Model file for the job. Use its own axes, mm. A direction names the side the tool comes from. Coordinates: 2 decimals unless noted, no trailing zeros. Order: outer loops, then holes, each group sorted by start corner. A loop starts at its lowest first (then second) coordinate and runs counter-clockwise, first axis right, second up. Notation, with made-up numbers: (37.5, -11.75) -> (88.5, -11.75) arc R4 ccw to (88.5, -7.75) -> close; hole circle Ø9 at (13, -39). An arc over 180 degrees is marked (long way). Write item = value, one per line. Start each with the question number.
Q1. Flat gauge pins, fed straight in: pin 1 (10 mm diameter, centred on y = -6.5, z = -9, fed in from -X); pin 2 (7.5 mm diameter, centred on x = -20, y = -11, fed in from -Z); pin 3 (9 mm diameter, centred on x = 3.5, y = -40, fed in from +Z). Where does each tip first touch, or does it go through?
Q2. Cut at B-B, the plane y = -33.5. List the corners of the cut face in (x, z) (1 decimal), plus the area to 3 significant figures.
Q3. 3-axis set-ups, long thin cutter, end or side, ignore diameter. For faces 1 (the face through (6.797, -33.859, 9.633)), 2 (the face through (-17.325, -1.141, 24.203)), 3 (the face through (-18, -17, 23)), 4 (the face through (-17.325, -33.859, 24.203)), 5 (the face through (1.203, -33.859, 8.874)): which of +Z, -Z, +X, -X, +Y, -Y reach the whole face in a straight line?
Q4. Wall check: line 1 (Z direction, x = -17, y = -15); line 2 (X direction, y = -4, z = -9); line 3 (Y direction, x = -17.5, z = 27). Give the ranges that are in metal, low to high. Write a range as from..to.
Q5. Cut at D-D, the plane y = -19. List the corners of the cut face in (x, z), plus the area to 3 significant figures.
from build123d import *

# Parameters (mm, degrees)
F1_DEPTH = 35
F3_DEPTH = 8
F4_R     = 5
F5_R     = 12
F6_R     = 3.99999
F7_R     = 3.99999


# Not quite as in the source:
# - a fillet or chamfer is up to 0.001 mm smaller than in the source, because OpenCascade refuses the exact size


with BuildPart() as f1:
    # F0 (on Front) → F1 (new body)
    with BuildSketch(Plane.XZ):
        Polygon((-30, 31), (-30, 23), (0, 23), (0, 0), (8, 0), (8, 31), align=None)
    extrude(amount=F1_DEPTH)

    # F2 (on Right) → F3 (join)
    with BuildSketch(Plane.YZ):
        Polygon((0, 0), (-50.1344501972, 0), (0, -18.2474475831), align=None)
    extrude(amount=F3_DEPTH)

    # F4
    f4_edges = [f1.edges().sort_by_distance(p)[0] for p in [
        (0, -17.5, 23),
    ]]
    fillet(f4_edges, radius=F4_R)

    # F5
    f5_edges = [f1.edges().sort_by_distance(p)[0] for p in [
        (8, -17.5, 31),
    ]]
    fillet(f5_edges, radius=F5_R)

    # F6 (radius 4 in the source; OpenCascade refuses exactly that, so slightly less here)
    f6_edges = [f1.edges().sort_by_distance(p)[0] for p in [
        (-17, -35, 31),
        (-17.5, -35, 23),
        (4.485281, -35, 27.485281),
        (-1.464466, -35, 21.535534),
        (0, -35, 9),
        (8, -35, 9.5),
    ]]
    fillet(f6_edges, radius=F6_R)

    # F7 (radius 4 in the source; OpenCascade refuses exactly that, so slightly less here)
    f7_edges = [f1.edges().sort_by_distance(p)[0] for p in [
        (-17, 0, 31),
        (-17.5, 0, 23),
        (0, 0, -0.123724),
        (8, 0, 0.376276),
        (4.485281, 0, 27.485281),
        (-1.464466, 0, 21.535534),
    ]]
    fillet(f7_edges, radius=F7_R)


solid = f1.part
Here are the results:
q1.pin_1 = 0
q1.pin_2 = 23
q1.pin_3 = 0
q2.outline = (-30, 23.9) -> (-5, 23.9) arc R5.9 cw to (0.9, 18) -> (0.9, 0) -> (0, 0) -> (0, -6.1) -> (8, -6.1) -> (8, 0) -> (7.1, 0) -> (7.1, 19) arc R11.1 ccw to (-4, 30.1) -> (-30, 30.1) -> close
q2.area = 410 mm²
q3.face_1 = +Z, +X, -Y
q3.face_2 = -Z, -X, +Y
q3.face_3 = -Z, -X, +Y, -Y
q3.face_4 = -Z, -X, -Y
q3.face_5 = -X, -Y
q4.line_1 = 23..31
q4.line_2 = 0..8
q4.line_3 = -35..0
q5.outline = (-30, 23) -> (-5, 23) arc R5 cw to (0, 18) -> (0, -11.33) -> (8, -11.33) -> (8, 19) arc R12 ccw to (-4, 31) -> (-30, 31) -> close
q5.area = 553 mm²
